Build history of the part. All positions in model axes, mm. A direction names the side the tool comes from. Coordinates: 2 decimals unless noted, no trailing zeros. Order: outer loops, then holes, each group sorted by start corner. A loop starts at its lowest first (then second) coordinate and runs counter-clockwise, first axis right, second up. Notation, with made-up numbers: (6, 83.5) - (65, 83.5) arc R32 ccw to (65, 122.5) - close; hole circle Ø3 at (78, 46.25). An arc over 180 degrees is marked (long way). Return JSON: item names as keys, results as strings.
from build123d import *

# Parameters (mm, degrees)
F0_R     = 88.9
F0_R_2   = 76.2
F1_DEPTH = 12.7
F3_DEPTH = 12.7
F4_W     = 12.015413
F4_H     = 48.26
F5_DEPTH = 12.7


with BuildPart() as f1:
    # F0 (on Top) → F1 (new body)
    with BuildSketch(Plane.XY):
        Circle(F0_R)
        Circle(F0_R_2, mode=Mode.SUBTRACT)
    extrude(amount=F1_DEPTH)

    # F2 (on face) → F3 (join)
    with BuildSketch(Plane(origin=(0, 0, 0), x_dir=(1, 0, 0), z_dir=(0, 0, -1))):
        with BuildLine():
            Line((-96.710376, 46.583939), (-82.060736, 34.194234))
            ThreePointArc((-82.060736, 34.194234), (-59.732506, 61.256656), (-32.116206, 82.896075))
            Line((-32.116206, 82.896075), (-40.030304, 92.636503))
            Line((-40.030304, 92.636503), (-96.710376, 46.583939))
        make_face()
    extrude(amount=-F3_DEPTH)

    # F4 (on face) → F5 (join)
    with BuildSketch(Plane(origin=(-61.255331, -75.391167, 0), x_dir=(0.776114, -0.630593, 0), z_dir=(-0.630593, -0.776114, 0))):
        with Locations((-1.727114, 6.35)):
            Rectangle(F4_W, F4_H)
    extrude(amount=-F5_DEPTH)


solid = f1.part
1. Probe L1, parallel to Y at x = 0, z = 5.75; L2, parallel to Z at x = 63, y = -57; L3, parallel to Y at x = 68, z = 6. List the from-to ranges inside material, lowest first.
Check values:
{"L1": "-88.9 to -76.2, 76.2 to 88.9", "L2": "0 to 12.7", "L3": "-57.26 to -34.39, 34.39 to 57.26"}
2. Cut at A-A on x = 0. Give the cut face in (y, z).
Check values:
{"outline": "(-88.9, 0) - (-76.2, 0) - (-76.2, 12.7) - (-88.9, 12.7) - close; (76.2, 0) - (88.9, 0) - (88.9, 12.7) - (76.2, 12.7) - close"}
3. Cut at C-C on z = 15. Give the cut face in (x, y), plus the area to 3 significant figures.
Check values:
{"outline": "(-67.26, -70.51) - (-57.93, -78.09) - (-49.92, -68.23) - (-59.25, -60.66) - close", "area": "153 mm²"}
4. Cut at D-D on y = -63. Give the cut face in (x, z), plus the area to 3 significant figures.
Check values:
{"outline": "(-76.51, 0) - (-61.15, 0) - (-61.15, -17.78) - (-56.37, -17.78) - (-56.37, 0) - (-42.87, 0) - (-42.87, 12.7) - (-56.37, 12.7) - (-56.37, 30.48) - (-61.15, 30.48) - (-61.15, 12.7) - (-76.51, 12.7) - close; (42.87, 0) - (62.72, 0) - (62.72, 12.7) - (42.87, 12.7) - close", "area": "850 mm²"}
5. Mould opens along Y. For faces 1 (the flat face through (-53.985, -73.231, 16.737)), 2 (the flat face through (-54.653, -64.392, 21.714)), 3 (the flat face through (-89.49, -40.48, 6.26)) say: pulls with the +Y half, pulls with the -Y half, needs draft (parallel to the pull), parting line crosses it, or undercut.
Check values:
{"face 1": "pulls with the -Y half", "face 2": "pulls with the +Y half", "face 3": "undercut"}
6. Tool access for faces 4 (the flat face through (-63.31, -65.654, 21.466)), 5 (the flat face through (-63.31, -65.654, -9.014)), 6 (the flat face through (-54.653, -64.392, -8.766)): list every direction of +Z, -Z, +X, -X, +Y, -Y with a clear straight run to the whole face (end or side of a thin tool).
Check values:
{"face 4": "+Z, -X, +Y", "face 5": "-Z, -X, +Y", "face 6": "-Z, +X, +Y"}
7. Drop flat-ended pins along their axis: pin 1 (1.5 mm diameter, centred on x = 64, y = -61, fed in from +Z); pin 2 (1 mm diameter, centred on x = -17, z = 3.5, fed in from -Y); pin 3 (5 mm diameter, centred on y = -65, z = 14.5, fed in from -X); pin 4 (3 mm diameter, centred on x = -34.5, z = -3, fed in from -Y). Give the stop position or say it passes through.
Check values:
{"pin 1": "z = 12.7", "pin 2": "y = -87.36", "pin 3": "x = -76.18", "pin 4": "through"}
